from build123d import *

# Parameters (mm, degrees)
MODEL_W                  = 43
MODEL_H                  = 90
MODEL_R                  = 2.05
EXTRUDE_1_DEPTH          = 21.8
FILLET_1_R               = 3
CUT_EXTRUDE_1_DEPTH      = 103.099167479
CUT_EXTRUDE_1_DEPTH_BACK = 103.099167479
FILLET_2_R               = 2.5
SKETCH_3_R               = 7.5
CUT_EXTRUDE_2_DEPTH      = 103.099167543
SKETCH_3_6_R             = 1.5
CUT_EXTRUDE_5_DEPTH      = 18
SKETCH_8_R               = 1.5
CUT_EXTRUDE_7_DEPTH      = 6
CHAMFER_3_SIZE           = 0.25
CHAMFER_4_SIZE           = 0.25


with BuildPart() as part:
    # Model → Бобышка-Вытянуть1 (new body)
    with BuildSketch(Plane.XY):
        with Locations((21.5, 45)):
            Rectangle(MODEL_W, MODEL_H)
        with Locations((10.05, 52.85)):
            Circle(MODEL_R, mode=Mode.SUBTRACT)
        with Locations((36.85, 52.85)):
            Circle(MODEL_R, mode=Mode.SUBTRACT)
        Polygon((14.5, 49), (14.5, 68), (34, 68), (34, 49), (39.5, 49), (39.5, 20), (3.5, 20), (3.5, 49), align=None, mode=Mode.SUBTRACT)
    extrude(amount=EXTRUDE_1_DEPTH)

    # Скругление1
    fillet_1_edges = [part.edges().sort_by_distance(p)[0] for p in [
        (3.5, 49, 10.9),
        (3.5, 20, 10.9),
        (39.5, 20, 10.9),
        (39.5, 49, 10.9),
        (34, 68, 10.9),
        (14.5, 68, 10.9),
    ]]
    fillet(fillet_1_edges, radius=FILLET_1_R)

    # Эскиз2 → Вырез-Вытянуть1 (cut, two sides: drawn at the far end of the back side and taken through both)
    with BuildSketch(Plane(origin=(43, 0, 0), x_dir=(0, 0, -1), z_dir=(1, 0, 0)).offset(-CUT_EXTRUDE_1_DEPTH_BACK)):
        Polygon((156.632056522, 70), (0, 70), (-15.8, 70), (-15.8, 20), (0, 20), (156.632056522, 20), (469.896169567, 20), (469.896169567, 70), align=None)
    extrude(amount=CUT_EXTRUDE_1_DEPTH + CUT_EXTRUDE_1_DEPTH_BACK, mode=Mode.SUBTRACT)

    # Скругление2
    fillet_2_edges = [part.edges().sort_by_distance(p)[0] for p in [
        (21.5, 70, 15.8),
        (3.25, 20, 15.8),
        (39.75, 20, 15.8),
    ]]
    fillet(fillet_2_edges, radius=FILLET_2_R - 0.0001)  # a hair under: the kernel refuses the full size

    # Эскиз3 → Вырез-Вытянуть2 (cut, through all)
    with BuildSketch(Plane(origin=(43, 0, 0), x_dir=(0, 0, -1), z_dir=(1, 0, 0))):
        with Locations(Location((-9.8, 80, 0), (0, 0, 90))):
            Circle(SKETCH_3_R)
        with Locations(Location((-9.8, 10, 0), (0, 0, 90))):
            Circle(SKETCH_3_R)
    extrude(amount=-CUT_EXTRUDE_2_DEPTH, mode=Mode.SUBTRACT)

    # Эскиз3<6> → Вырез-Вытянуть5 (cut)
    with BuildSketch(Plane(origin=(43, 0, 0), x_dir=(0, 0, -1), z_dir=(1, 0, 0))):
        with Locations(Location((-18.8, 86.5, 0), (0, 0, 90))):
            Circle(SKETCH_3_6_R)
        with Locations(Location((-18.8, 69.4, 0), (0, 0, 90))):
            Circle(SKETCH_3_6_R)
    extrude(amount=-CUT_EXTRUDE_5_DEPTH, mode=Mode.SUBTRACT)

    # Эскиз8 → Вырез-Вытянуть7 (cut)
    with BuildSketch(Plane(origin=(0, 0, 0), x_dir=(-1, 0, 0), z_dir=(0, 0, -1))):
        with Locations((-35, 86.5)):
            Circle(SKETCH_8_R)
        with Locations(Location((-8, 86.5, 0), (0, 0, 358.703677977))):
            Circle(SKETCH_8_R)
        with Locations((-8, 3.5)):
            Circle(SKETCH_8_R)
        with Locations(Location((-35, 3.5, 0), (0, 0, 1.296322023))):
            Circle(SKETCH_8_R)
    extrude(amount=-CUT_EXTRUDE_7_DEPTH, mode=Mode.SUBTRACT)

    # Фаска3
    chamfer_3_edges = [part.edges().sort_by_distance(p)[0] for p in [
        (43, 80, 0),
        (43, 70, 6.65005),
        (0, 10, 0),
        (0, 20, 6.65005),
        (21.5, 70, 0),
        (0, 70, 6.65005),
        (43, 45, 21.8),
        (0, 45, 15.8),
        (43, 45, 15.8),
        (43, 20, 6.65005),
        (0, 69.267796242, 15.067796242),
        (43, 69.267796242, 15.067796242),
        (43, 20.732203758, 15.067796242),
        (0, 20.732203758, 15.067796242),
        (43, 2.5, 9.8),
        (0, 2.5, 9.8),
        (0, 72.5, 9.8),
        (43, 72.5, 9.8),
        (43, 85, 18.8),
        (43, 67.9, 18.8),
        (36.5, 86.5, 0),
        (9.499616095, 86.533934736, 0),
        (9.5, 3.5, 0),
        (36.499616095, 3.466065264, 0),
        (43, 10, 0),
        (21.5, 0, 0),
        (21.5, 20, 0),
        (0, 80, 0),
        (21.5, 90, 0),
        (0, 45, 21.8),
        (43, 90, 10.9),
        (43, 0, 10.9),
        (0, 0, 10.9),
        (0, 90, 10.9),
    ]]
    chamfer(chamfer_3_edges, length=CHAMFER_3_SIZE)

    # Фаска4
    chamfer_4_edges = [part.edges().sort_by_distance(p)[0] for p in [
        (21.5, 90, 21.8),
        (21.5, 0, 21.8),
    ]]
    chamfer(chamfer_4_edges, length=CHAMFER_4_SIZE)


solid = part.part
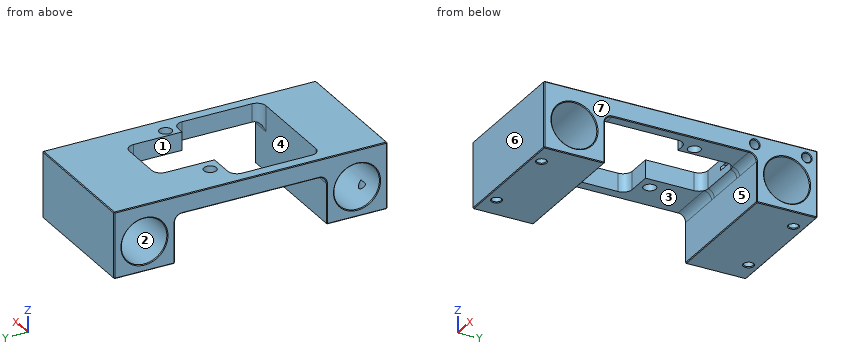
The listing builds one solid part. Answer for the finished solid, in the listing's coordinates (mm). Face numbers are marked on the shaded views. A direction names the side the tool comes from. Coordinates: 2 decimals unless noted, no trailing zeros. Loops run counter-clockwise (first coordinate to the right, second up) from the corner with the lowest first, then second, coordinate; pieces in that order, holes last.
1) Determine the mould class of the marked faces 5, 6 and 7 for opening direction Y: pulls with the +Y half, pulls with the -Y half, needs draft (parallel to the pull), parting line crosses it, or undercut.
2) Find section B-B on z = 9.8. Give the number of separate pieces and of enclosed holes in the cut face, then the cut area to 4 significant figures.
3) A tool of negligible diameter and unlimited length cuts with its end or side. For the marked faces 1, 2, 3 and 4, from which of +Z, -Z, +X, -X, +Y, -Y can it reach the whole face along a straight path? Write none if from no direction.
4) Find the intervals of material crossed by L1, parallel to X at y = 3.5, z = 2; L2, parallel to Y at x = 12.5, z = 9.75; L3, parallel to Y at x = 35, z = 19.25, in increasing order.
5) Find section A-A on y = 44. Write down the section's boundary in (x, z), then the cut area to 3 significant figures.
6) Flat-ended cylindrical pins translate along their axes: pin 1 Ø3 at (y, z) = (25.5, 15) entering from +X; pin 2 Ø1.2 at (x, y) = (8, 3) entering from -Z; pin 3 Ø1.5 at (y, z) = (69, 19) entering from +X; pin 4 Ø11 at (x, y) = (37.5, 38) entering from -Z. Find the tip coordinate at first contact, or state that the pin passes through.
7) Find section D-D on y = 54. Write down the section's boundary in (x, z), then the cut area to 3 significant figures.
Values:
1. face 5: undercut
1. face 6: pulls with the -Y half
1. face 7: needs draft
2. separate pieces: 4
2. enclosed holes: 0
2. area: 429.5 mm2
3. face 1: +Z, -Z
3. face 2: +X, -X
3. face 3: -Z, +X, -X
3. face 4: -Z
4. L1: x = 0 to 6.5, 9.5 to 33.5, 36.5 to 43
4. L2: y = 0 to 2.5, 17.5 to 20, 70 to 72.5, 87.5 to 90
4. L3: y = 0 to 20, 49 to 51.97, 53.73 to 67.97, 70.83 to 85.07, 87.93 to 90
5. outline: (0, 16.05) - (0.25, 15.8) - (3.5, 15.8) - (3.5, 21.8) - (0.25, 21.8) - (0, 21.55) - close; (39.5, 15.8) - (42.75, 15.8) - (43, 16.05) - (43, 21.55) - (42.75, 21.8) - (39.5, 21.8) - close
5. area: 41.9 mm2
6. pin 1: stops at x = 43
6. pin 2: stops at z = 6
6. pin 3: stops at x = 25
6. pin 4: stops at z = 15.8
7. outline: (0, 16.05) - (0.25, 15.8) - (8.35, 15.8) - (8.35, 21.8) - (0.25, 21.8) - (0, 21.55) - close; (11.75, 15.8) - (14.5, 15.8) - (14.5, 21.8) - (11.75, 21.8) - close; (34, 15.8) - (35.15, 15.8) - (35.15, 21.8) - (34, 21.8) - close; (38.55, 15.8) - (42.75, 15.8) - (43, 16.05) - (43, 21.55) - (42.75, 21.8) - (38.55, 21.8) - close
7. area: 100 mm2
